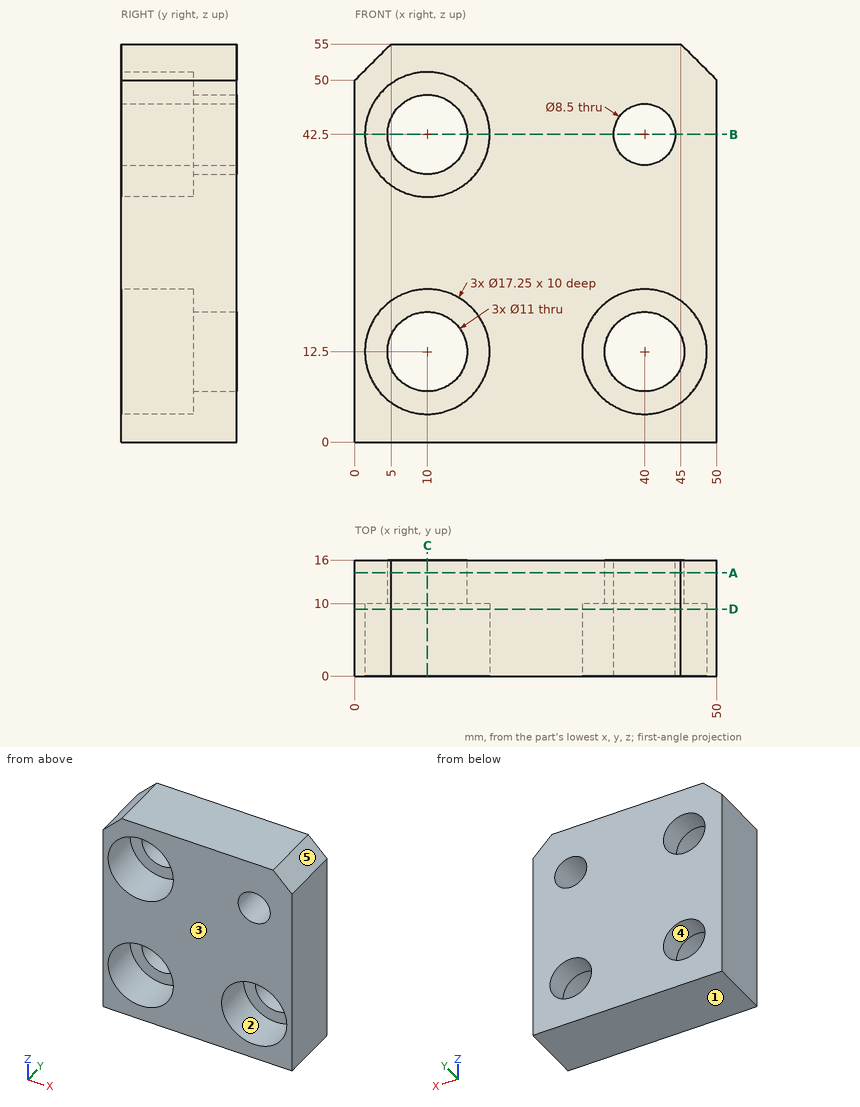
Source: three-view drawing plus pictorial views. Frame: mm from the lowest corner of the part. A direction names the side the tool comes from. Give positions to 0.01 mm unless a question says otherwise; leave off trailing zeros. Order: outer loops, then holes, each group sorted by start corner. A loop starts at its lowest first (then second) coordinate and runs counter-clockwise, first axis right, second up. Notation, with made-up numbers: (56, -14) - (84, -14) arc R24 ccw to (84, -1) - close; hole circle Ø1 at (78.5, 77.25). An arc over 180 degrees is marked (long way). Answer as a JSON object with one key per item and string values. Group by question number.
Q1. Cut plane A-A, the plane y = 14.25. Output: boundary loops of the cut face in (x, z).
Q2. Line query: probe 1 along Z at (x, y) = (10, 13.85); probe 2 along Z at (x, y) = (40, 4) (3 decimals); probe 3 along X at (y, z) = (9.5, 14). Output: solid intervals per line, ascending.
Q3. Cut plane D-D, the plane y = 9.25. Output: boundary loops of the cut face in (x, z) (3 decimals), then the cut area to 3 significant figures.
Q4. Mould query, pull axis Z, two halves, no side actions, for the marked faces 3, 4 and 5. Classes: pulls with the +Z half, pulls with the -Z half, needs draft (parallel to the pull), parting line crosses it, or undercut.
Q5. Cut plane B-B, the plane z = 42.5. Output: boundary loops of the cut face in (x, y) (3 decimals), then the cut area to 4 significant figures.
Q6. Set-up query: the marked faces 1 and 2. Return all of +Z, -Z, +X, -X, +Y, -Y with unobstructed straight access to the full face (end or side cutting, diameter ignored); none if empty.
Q7. Cut plane C-C, the plane x = 10. Output: boundary loops of the cut face in (y, z) (3 decimals).
Q8. First-contact query: pin 1 Ø10.5 at (x, z) = (40, 12.5) entering from +Y. Flat tip, straight axial feed; report the tip coordinate or a pass-through.
Results:
{
 "1": {"outline": "(0, 0) - (50, 0) - (50, 50) - (45, 55) - (5, 55) - (0, 50) - close; hole circle Ø11 at (10, 12.5); hole circle Ø11 at (10, 42.5); hole circle Ø11 at (40, 12.5); hole circle Ø8.5 at (40, 42.5)"},
 "2": {"probe 1": "0 to 7, 18 to 37, 48 to 55", "probe 2": "0 to 3.875, 21.125 to 38.25, 46.75 to 55", "probe 3": "0 to 1.51, 18.49 to 31.51, 48.49 to 50"},
 "3": {"outline": "(0, 0) - (50, 0) - (50, 50) - (45, 55) - (5, 55) - (0, 50) - close; hole circle Ø17.25 at (10, 12.5); hole circle Ø17.25 at (10, 42.5); hole circle Ø17.25 at (40, 12.5); hole circle Ø8.5 at (40, 42.5)", "area": "1,970 mm^2"},
 "4": {"face 3": "needs draft", "face 4": "undercut", "face 5": "pulls with the +Z half"},
 "5": {"outline": "(0, 0) - (1.375, 0) - (1.375, 10) - (4.5, 10) - (4.5, 16) - (0, 16) - close; (15.5, 10) - (18.625, 10) - (18.625, 0) - (35.75, 0) - (35.75, 16) - (15.5, 16) - close; (44.25, 0) - (50, 0) - (50, 16) - (44.25, 16) - close", "area": "425.5 mm^2"},
 "6": {"face 1": "-Z, +X, -X, +Y, -Y", "face 2": "-Y"},
 "7": {"outline": "(0, 0) - (16, 0) - (16, 7) - (10, 7) - (10, 3.875) - (0, 3.875) - close; (0, 21.125) - (10, 21.125) - (10, 18) - (16, 18) - (16, 37) - (10, 37) - (10, 33.875) - (0, 33.875) - close; (0, 51.125) - (10, 51.125) - (10, 48) - (16, 48) - (16, 55) - (0, 55) - close"},
 "8": {"pin 1": "through"}
}
